Could you check a few things on this model? Use its own coordinates, in mm. Face numbers are marked on the shaded views. A direction names the side the tool comes from. Give positions to 0.01 mm unless a question says otherwise; leave off trailing zeros. Order: outer loops, then holes, each group sorted by start corner. A loop starts at its lowest first (then second) coordinate and runs counter-clockwise, first axis right, second up. Notation, with made-up numbers: (12.5, 41) -> (46.5, 41) arc R18 cw to (46.5, 51) -> close; hole circle Ø3 at (12.25, 20). An arc over 180 degrees is marked (long way). One line per item, written item: value.
```python
from build123d import *

# Parameters (mm, degrees)
F0_R     = 17.65
F0_R_2   = 1.05
F0_W     = 17.6
F0_H     = 28
F1_DEPTH = 4.1
F2_W     = 8.4405994534
F2_H     = 9.594688829
F2_W_2   = 9.8450831422
F2_H_2   = 12.0924381804
F2_W_3   = 11.2190096889
F2_H_3   = 12.7369980328
F2_W_4   = 11.1257450883
F3_DEPTH = 4.101
F4_R     = 1
F5_DEPTH = 30.451


with BuildPart() as f1:
    # F0 (on Top) → F1 (new body)
    with BuildSketch(Plane.XY):
        Circle(F0_R)
        with Locations((0, -15.5)):
            Circle(F0_R_2, mode=Mode.SUBTRACT)
        with Locations((-15.5, 0)):
            Circle(F0_R_2, mode=Mode.SUBTRACT)
        Rectangle(F0_W, F0_H, mode=Mode.SUBTRACT)
        with Locations((15.5, 0)):
            Circle(F0_R_2, mode=Mode.SUBTRACT)
        with Locations((0, 15.5)):
            Circle(F0_R_2, mode=Mode.SUBTRACT)
    extrude(amount=F1_DEPTH)

    # F2 (on face) → F3 (cut, through all)
    with BuildSketch(Plane.XY.offset(4.1)):
        with Locations((-17.0202997267, 10.7973444145)):
            Rectangle(F2_W, F2_H)
        with Locations((17.7225415711, 12.0462190902)):
            Rectangle(F2_W_2, F2_H_2)
        with Locations((18.4095048444, -12.3684990164)):
            Rectangle(F2_W_3, F2_H_3)
        with Locations((-18.3628725441, -12.3684990164)):
            Rectangle(F2_W_4, F2_H_3)
    extrude(amount=-F3_DEPTH, mode=Mode.SUBTRACT)

    # F4 (on face) → F5 (cut, through all)
    with BuildSketch(Plane(origin=(-12.8, 0, 0), x_dir=(0, -1, 0), z_dir=(-1, 0, 0))):
        with Locations((-8.5, 2.05)):
            Circle(F4_R)
        with Locations((8.5, 2.05)):
            Circle(F4_R)
    extrude(amount=-F5_DEPTH, mode=Mode.SUBTRACT)


solid = f1.part
```
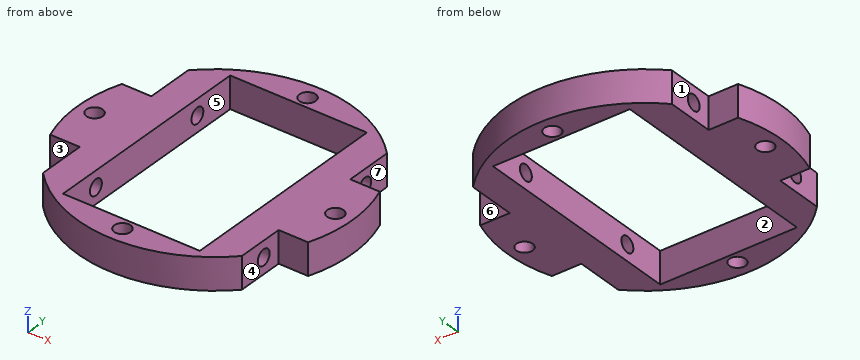
1) Suppose I cut it at A-A, the plane x = -15.5. Write out the boundary of the cut face in (y, z).
Answer below:
outline: (-6, 0) -> (-1.05, 0) -> (-1.05, 4.1) -> (-6, 4.1) -> close; (1.05, 0) -> (6, 0) -> (6, 4.1) -> (1.05, 4.1) -> close
2) If I drill on line 1 along X through (y, z) = (-9, 0.75); line 2 along Z through (x, y) = (10.1, 8.5); line 3 along Y through (x, z) = (11.5, 2.6), over which ranges is the centre line in solid material (lowest first)?
Answer below:
line 1: x = -12.8 to -8.8, 8.8 to 12.8
line 2: z = 0 to 1.05, 3.05 to 4.1
line 3: y = -13.39 to -9.34, -7.66 to 7.66, 9.34 to 13.39
3) For the marked faces 1, 2, 3 and 4, which set-ups out of +Z, -Z, +X, -X, +Y, -Y let a thin tool reach every point of the face, with its end or its side?
Answer below:
face 1: +Z, -Z, -X, +Y
face 2: +Z, -Z
face 3: +Z, -Z, -X, -Y
face 4: +Z, -Z, +X, -Y
4) Suppose I cut it at D-D, the plane z = 3.65. Write out the boundary of the cut face in (x, y), then the cut area to 3 significant figures.
Answer below:
outline: (-16.6, -6) -> (-12.8, -6) -> (-12.8, -12.15) arc R17.65 ccw to (12.8, -12.15) -> (12.8, -6) -> (16.6, -6) arc R17.65 ccw to (16.6, 6) -> (12.8, 6) -> (12.8, 12.15) arc R17.65 ccw to (-12.8, 12.15) -> (-12.8, 6) -> (-16.6, 6) arc R17.65 ccw to start; hole circle Ø2.1 at (-15.5, 0); hole (-8.8, -14) -> (8.8, -14) -> (8.8, 14) -> (-8.8, 14) -> close; hole circle Ø2.1 at (0, -15.5); hole circle Ø2.1 at (0, 15.5); hole circle Ø2.1 at (15.5, 0)
area: 418 mm2
5) We'd pull the mould along X, two halves only. Please class the marked faces 5, 6 and 7: +X half, -X half, draft (parallel to the pull), parting line (faces both ways), or undercut.
Answer below:
face 5: undercut
face 6: draft
face 7: +X half
6) Suppose I cut it at C-C, the plane y = 0. Write out the boundary of the cut face in (x, z), then the cut area to 4 significant figures.
Answer below:
outline: (-17.65, 0) -> (-16.55, 0) -> (-16.55, 4.1) -> (-17.65, 4.1) -> close; (-14.45, 0) -> (-8.8, 0) -> (-8.8, 4.1) -> (-14.45, 4.1) -> close; (8.8, 0) -> (14.45, 0) -> (14.45, 4.1) -> (8.8, 4.1) -> close; (16.55, 0) -> (17.65, 0) -> (17.65, 4.1) -> (16.55, 4.1) -> close
area: 55.35 mm2
7) For P1, Ø2, axis at y = 8, z = 2.5, coming from the +X side; P2, Ø2, axis at y = -1.5, z = 3, coming from the -X side; P3, Ø1.9, axis at x = 14.5, z = 1, coming from the +Y side, each with a flat end and sliding along its axis, tell me the tip position at first contact or that it passes through.
Answer below:
P1: stops at x = 12.8
P2: stops at x = -17.64
P3: stops at y = 6
8) Suppose I cut it at B-B, the plane x = 0. Write out the boundary of the cut face in (y, z).
Answer below:
outline: (-17.65, 0) -> (-16.55, 0) -> (-16.55, 4.1) -> (-17.65, 4.1) -> close; (-14.45, 0) -> (-14, 0) -> (-14, 4.1) -> (-14.45, 4.1) -> close; (14, 0) -> (14.45, 0) -> (14.45, 4.1) -> (14, 4.1) -> close; (16.55, 0) -> (17.65, 0) -> (17.65, 4.1) -> (16.55, 4.1) -> close
